Verification items for this drawing (mm, ordinates from the low corner). Round coordinates to 2 decimals unless told otherwise and drop trailing zeros. Order: outer loops, then holes, each group sorted by start corner. A loop starts at its lowest first (then second) coordinate and runs counter-clockwise, first axis right, second up. Notation, with made-up numbers: (8.25, 2.5) -> (27.25, 2.5) arc R7 cw to (27.25, 7.5) -> close; hole circle Ø10 at (35, -4.75). An arc over 180 degrees is marked (long way). Use a Markdown table: item, result. Add a question column.
Item 1: Sectioned sample at A-A, the plane x = 10. Record the cut outline in (y, z).
Item 2: Sectioned sample at C-C, the plane z = 37. Record the cut outline in (x, y).
Item 3: Gauge pin test, flat ends, axial feed: pin 1 Ø1.5 at (y, z) = (1, 2) entering from +X; pin 2 Ø0.9 at (x, y) = (17.5, 1) entering from +Z. Record the tip position at first contact, or that the pin passes through.
Item 4: Sectioned sample at B-B, the plane z = 61.5. Record the cut outline in (x, y).
Item 5: Sectioned sample at D-D, the plane y = 1.6. State how many separate pieces and enclosed holes the cut face has, and give its area (3 significant figures).
Item 6: Material ranges on probe 1 along Z at (x, y) = (5, 1.6); probe 2 along X at (y, z) = (1, 37); probe 3 along Z at (x, y) = (9.75, 2.3), recorded low to high. Write a range as [from, to].
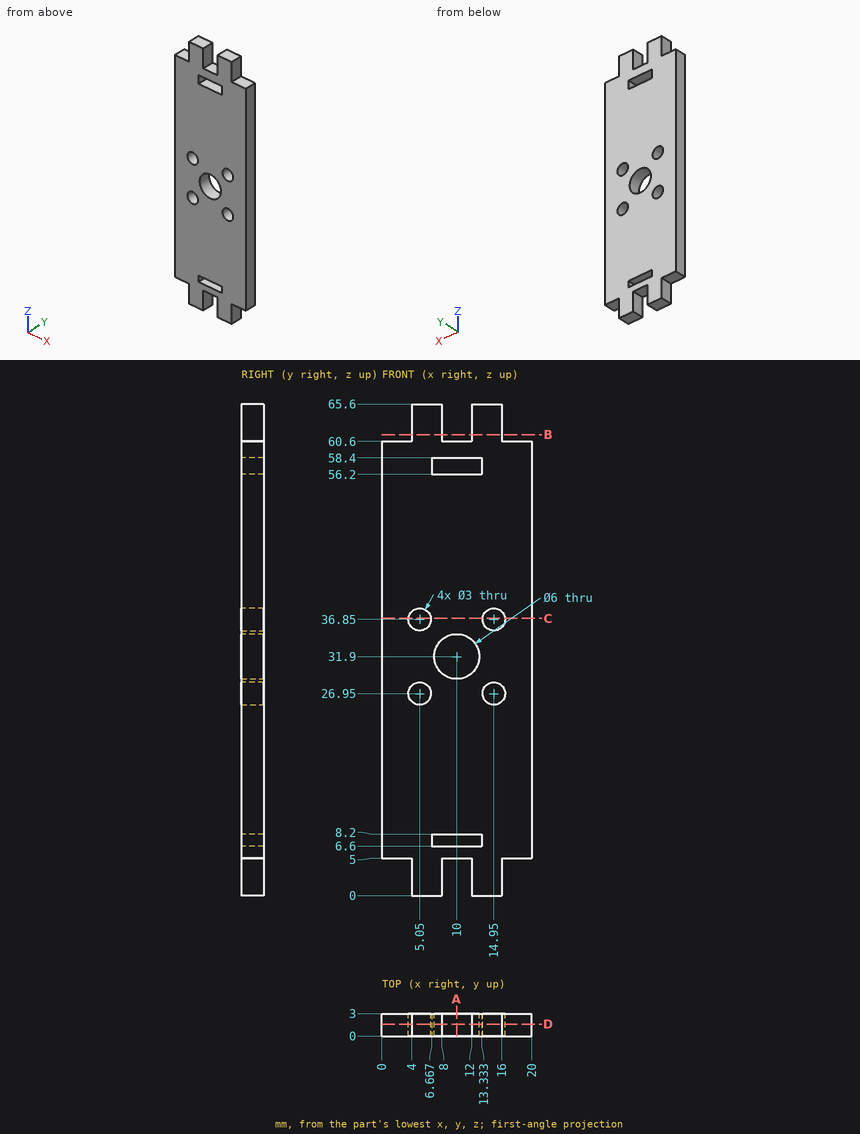
Found:
| question | item | result |
|---|---|---|
| 1 | outline | (0, 5) -> (3, 5) -> (3, 6.6) -> (0, 6.6) -> close; (0, 8.2) -> (3, 8.2) -> (3, 28.9) -> (0, 28.9) -> close; (0, 34.9) -> (3, 34.9) -> (3, 56.2) -> (0, 56.2) -> close; (0, 58.4) -> (3, 58.4) -> (3, 60.6) -> (0, 60.6) -> close |
| 2 | outline | (0, 0) -> (3.56, 0) -> (3.56, 3) -> (0, 3) -> close; (6.54, 0) -> (13.46, 0) -> (13.46, 3) -> (6.54, 3) -> close; (16.44, 0) -> (20, 0) -> (20, 3) -> (16.44, 3) -> close |
| 3 | pin 1 | stops at x = 16 |
| 3 | pin 2 | stops at z = 60.6 |
| 4 | outline | (4, 0) -> (8, 0) -> (8, 3) -> (4, 3) -> close; (12, 0) -> (16, 0) -> (16, 3) -> (12, 3) -> close |
| 5 | separate pieces | 1 |
| 5 | enclosed holes | 7 |
| 5 | area | 1,110 mm2 |
| 6 | probe 1 | z = [0, 25.45], [28.45, 35.35], [38.35, 65.6] |
| 6 | probe 2 | x = [0, 3.56], [6.54, 13.46], [16.44, 20] |
| 6 | probe 3 | z = [5, 6.6], [8.2, 28.91], [34.89, 56.2], [58.4, 60.6] |
